Could you check a few things on this model? Use its own coordinates, in mm. A direction names the side the tool comes from. Round coordinates to 2 decimals unless told otherwise and drop trailing zeros. Write each loop counter-clockwise with the first axis right and the second up, starting at its lowest first coordinate (ties: lowest second). Pieces come first, ordered by that corner, then holes. Notation, with made-up numbers: (50.25, 49.5) -> (96.25, 49.5) arc R10 ccw to (96.25, 57.5) -> close; hole circle Ø9 at (-16.5, 44). An arc over 180 degrees is marked (long way). Return JSON: item names as keys, results as strings.
Autodesk Inventor part; units mm, degrees
ref_plane "YZ Plane" through (0, 0, 0) normal (1, 0, 0) x (0, 1, 0)
ref_plane "XZ Plane" through (0, 0, 0) normal (0, 1, 0) x (-1, 0, 0)
ref_plane "XY Plane" through (0, 0, 0) normal (0, 0, 1) x (1, 0, 0)
sketch "Sketch1" plane through (0, 0, 0) normal (1, 0, 0) x (0, 1, 0)
  line L0 (0, 0) -> (69.85, 0)
  line L1 (69.85, 0) -> (69.85, -88.9)
  line L2 (69.85, -88.9) -> (0, -88.9)
  line L3 (0, -88.9) -> (0, 0)
  dimension "d0" = 88.9
  dimension "d1" = 69.85
extrude "Extrusion1" add sketch "Sketch1" along normal blind 152.4
sketch "Sketch4" plane through (152.4, 0, 0) normal (1, 0, 0) x (0, 0, -1)
  line L0 (88.9, 69.85) -> (0, 69.85)
  line L1 (25.4, 69.85) -> (63.5, 69.85)
  line L2 (63.5, 69.85) -> (63.5, 57.15)
  line L3 (63.5, 57.15) -> (25.4, 57.15)
  line L4 (25.4, 57.15) -> (25.4, 69.85)
  line L5 (88.9, 0) -> (88.9, 69.85)
  point P0 (0, 0)
  point P1 (63.5, 69.85)
  dimension "d6" = 38.1
  dimension "d7" = 25.4
  dimension "d8" = 12.7
extrude "Extrusion3" cut sketch "Sketch4" against normal through all
sketch "Sketch5" plane through (0, 0, 0) normal (0, 0, 1) x (1, 0, 0)
  line L0 (0, 69.85) -> (152.4, 69.85)
  line L1 (63.5, 69.85) -> (152.4, 25.4)
  line L2 (152.4, 69.85) -> (152.4, 0)
  line L3 (0, 69.85) -> (0, 0)
  line L4 (0, 0) -> (152.4, 0)
  line L5 (152.4, 69.85) -> (152.4, 0)
  line L6 (0, 69.85) -> (152.4, 69.85)
  dimension "d28" = 25.4
  dimension "d29" = 63.5
extrude "Extrusion4" cut sketch "Sketch5" against normal through all contours L0 L2 L1
sketch "Sketch6" plane through (0, 69.85, -63.5) normal (0, 1, 0) x (1, 0, 0)
  line L0 (152.4, 25.4) -> (152.4, -63.5)
  line L1 (152.4, -19.05) -> (101.6, -63.5)
  line L2 (0, -63.5) -> (152.4, -63.5)
  line L3 (0, 25.4) -> (0, -63.5)
  line L4 (0, 25.4) -> (0, -63.5)
  line L5 (0, 25.4) -> (152.4, 25.4)
  line L6 (63.5, 25.4) -> (152.4, 25.4)
  point P0 (0, -38.1)
  point P1 (0, 0)
  dimension "d22" = 101.6
  dimension "d30" = 44.45
extrude "Extrusion5" cut sketch "Sketch6" against normal through all contours L0 L2 L1
sketch "Sketch8" plane through (0, 0, 0) normal (0, 0, 1) x (1, 0, 0)
  line L0 (0, 69.85) -> (0, 0)
  line L1 (0, 0) -> (101.6, 0)
  point P0 (38.1, 31.75)
  dimension "d31" = 38.1
  dimension "d32" = 31.75
hole "Hole1" at (38.1, 31.75, 0) direction (0, 0, -1) diameter 25.4 end through all
properties part number "WedgeBlock"
1) Will these pins go through, and if not, where does the flat tip stop? pin 1 Ø1 at (x, y) = (103, 13) entering from +Z; pin 2 Ø3 at (y, z) = (14, -37.5) entering from +X; pin 3 Ø19 at (x, z) = (61, -53.5) entering from +Y.
Return value:
{"pin 1": "z = -0.79", "pin 2": "x = 146.17", "pin 3": "y = 57.15"}
2) I want a section at C-C, the plane y = 36.5. Please give me the cut outline in (x, z) (3 decimals).
Return value:
{"outline": "(0, -88.9) -> (26.322, -88.9) -> (26.322, 0) -> (0, 0) -> close; (49.878, -88.9) -> (130.2, -88.9) -> (130.2, -25.025) -> (101.6, 0) -> (49.878, 0) -> close"}
3) I want a section at B-B, the plane z = -71. Please give me the cut outline in (x, y), and give its area (3 significant figures).
Return value:
{"outline": "(0, 0) -> (152.4, 0) -> (152.4, 25.4) -> (63.5, 69.85) -> (0, 69.85) -> close; hole circle Ø25.4 at (38.1, 31.75)", "area": "8,160 mm²"}
4) I want a section at A-A, the plane x = 41.5. Please give me the cut outline in (y, z), and give its area (3 significant figures).
Return value:
{"outline": "(0, -88.9) -> (19.51, -88.9) -> (19.51, 0) -> (0, 0) -> close; (43.99, -88.9) -> (69.85, -88.9) -> (69.85, -63.5) -> (57.15, -63.5) -> (57.15, -25.4) -> (69.85, -25.4) -> (69.85, 0) -> (43.99, 0) -> close", "area": "3,550 mm²"}
5) Thinking about a two-plate mould opening in Y: for faces 3 (the face through (45, 57.15, -45)), 4 (the face through (50.5, 34.5, -45.1)), 5 (the face through (35, 63, -25.4)), which applies, pulls with the +Y half, pulls with the -Y half, needs draft (parallel to the pull), parting line crosses it, or undercut?
Return value:
{"face 3": "pulls with the +Y half", "face 4": "undercut", "face 5": "needs draft"}
6) If I drill on probe 1 along Y at (x, z) = (38, -57); probe 2 along Y at (x, z) = (38.1, -65); probe 3 along Z at (x, y) = (61.5, 62), over which ranges is the centre line in solid material (lowest first)? Write a range as [from, to].
Return value:
{"probe 1": "[0, 19.05], [44.45, 57.15]", "probe 2": "[0, 19.05], [44.45, 69.85]", "probe 3": "[-88.9, -63.5], [-25.4, 0]"}
7) I want a section at D-D, the plane x = 68. Please give me the cut outline in (y, z), and give its area (3 significant figures).
Return value:
{"outline": "(0, -88.9) -> (67.6, -88.9) -> (67.6, -63.5) -> (57.15, -63.5) -> (57.15, -25.4) -> (67.6, -25.4) -> (67.6, 0) -> (0, 0) -> close", "area": "5,610 mm²"}
8) For faces 1 (the face through (35, 64, -63.5)), 2 (the face through (31, 69.85, -13)), which set-ups out of +Z, -Z, +X, -X, +Y, -Y let a thin tool reach every point of the face, with its end or its side?
Return value:
{"face 1": "+X, -X, +Y", "face 2": "+Z, -Z, +X, -X, +Y"}
